Verification items for the finished model (mm, model axes). Give positions to 0.01 mm unless a question says otherwise; leave off trailing zeros. Order: outer loops, then holes, each group sorted by start corner. A loop starts at its lowest first (then second) coordinate and runs counter-clockwise, first axis right, second up. Notation, with made-up numbers: (49.25, 33.5) -> (93.25, 33.5) arc R16 ccw to (93.25, 56.5) -> close; hole circle Ø1 at (48.25, 10.25). An arc over 180 degrees is marked (long way). One line per question, with ' | ' between items. Start each with the question number.
Q1. Material ranges on probe 1 along X at (y, z) = (105.5, 3.5); probe 2 along Y at (x, z) = (-114.3, 5.75); probe 3 along X at (y, z) = (99, 3), recorded low to high. Write a range as [from, to].
Q2. Section check A-A on x = -114.3. Record the cut outline in (y, z), plus the area to 3 significant figures.
Q3. Section check C-C on x = -323.85. Record the cut outline in (y, z).
Q4. Go/stop test with flat-tipped pins: pin 1 (2 mm diameter, centred on x = -303, z = 4, fed in from +Y); pin 2 (1.5 mm diameter, centred on y = 137, z = 5.5, fed in from +X). Record where each tip stops, or that it passes through.
Q5. Section check B-B on y = 29. Record the cut outline in (x, z).
Q6. Mould release check, pull along Y, two halves, no side actions. Record for faces 1 (the cylindrical face through (-80.81, 158.52, 3.76)), 2 (the cylindrical face through (-366.55, 107.02, 3.76)), 3 (the flat face through (-50.57, 25.46, 3.76)): released by +Y, released by -Y, zero draft, split by the parting line, or undercut.
Q7. Section check D-D on z = 2.75. Give the number of separate pieces and of enclosed holes in the cut face, plus the area to 3 significant figures.
from build123d import *

# Parameters (mm, degrees)
SKETCH1_R           = 27.4955
SKETCH1_R_2         = 52.3875
SKETCH1_R_3         = 3.2512
SKETCH1_R_4         = 4.49961
BOSS_EXTRUDE1_DEPTH = 7.62


with BuildPart() as part:
    # Sketch1 → Boss-Extrude1 (new body)
    with BuildSketch(Plane.XY):
        with BuildLine():
            Line((-328.252358788, 147.362734983), (-120.623830303, 167.33652539))
            ThreePointArc((-120.623830303, 167.33652539), (-80.305183306, 158.218318925), (-53.30558743, 126.917251733))
            Line((-53.30558743, 126.917251733), (-9.46754648, 21.302488163))
            ThreePointArc((-9.46754648, 21.302488163), (-11.996916286, 10.47886003), (-23.061809086, 9.422079593))
            Line((-23.061809086, 9.422079593), (-78.866488962, 41.953179506))
            ThreePointArc((-78.866488962, 41.953179506), (-82.120777387, 42.89869406), (-85.437090509, 42.2012285))
            ThreePointArc((-85.437090509, 42.2012285), (-113.899521097, 35.561214301), (-142.440389403, 41.855543485))
            ThreePointArc((-142.440389403, 41.855543485), (-145.776424621, 42.51215325), (-149.027245523, 41.515945031))
            Line((-149.027245523, 41.515945031), (-223.676633484, -3.557736497))
            ThreePointArc((-223.676633484, -3.557736497), (-228.504182895, -4.928354428), (-233.358329437, -3.655134819))
            Line((-233.358329437, -3.655134819), (-346.816870084, 61.773732857))
            ThreePointArc((-346.816870084, 61.773732857), (-368.77925543, 111.345290274), (-328.252358788, 147.362734983))
        make_face()
        with Locations(Location((-323.85, 101.6, 0), (0, 0, 180))):
            Circle(SKETCH1_R, mode=Mode.SUBTRACT)
        with Locations(Location((-114.3, 101.6, 0), (0, 0, 180))):
            Circle(SKETCH1_R_2, mode=Mode.SUBTRACT)
        with Locations(Location((-228.6, 4.596163622, 0), (0, 0, 180))):
            Circle(SKETCH1_R_3, mode=Mode.SUBTRACT)
        with Locations(Location((-18.264817524, 17.65096147, 0), (0, 0, 180))):
            Circle(SKETCH1_R_3, mode=Mode.SUBTRACT)
        with Locations(Location((-323.85, 140.59916, 0), (0, 0, 180))):
            Circle(SKETCH1_R_4, mode=Mode.SUBTRACT)
        with Locations(Location((-298.781823164, 131.475089804, 0), (0, 0, 180))):
            Circle(SKETCH1_R_4, mode=Mode.SUBTRACT)
        with Locations(Location((-285.443324871, 108.372133065, 0), (0, 0, 180))):
            Circle(SKETCH1_R_4, mode=Mode.SUBTRACT)
        with Locations(Location((-290.075736714, 82.10042, 0), (0, 0, 180))):
            Circle(SKETCH1_R_4, mode=Mode.SUBTRACT)
        with Locations(Location((-310.511501707, 64.952777131, 0), (0, 0, 180))):
            Circle(SKETCH1_R_4, mode=Mode.SUBTRACT)
        with Locations(Location((-337.188498293, 64.952777131, 0), (0, 0, 180))):
            Circle(SKETCH1_R_4, mode=Mode.SUBTRACT)
        with Locations(Location((-357.624263286, 82.10042, 0), (0, 0, 180))):
            Circle(SKETCH1_R_4, mode=Mode.SUBTRACT)
        with Locations(Location((-362.256675129, 108.372133065, 0), (0, 0, 180))):
            Circle(SKETCH1_R_4, mode=Mode.SUBTRACT)
        with Locations(Location((-348.918176836, 131.475089804, 0), (0, 0, 180))):
            Circle(SKETCH1_R_4, mode=Mode.SUBTRACT)
    extrude(amount=BOSS_EXTRUDE1_DEPTH)


solid = part.part
Filled in:
1) probe 1: [-369.66, -365.72], [-358.79, -351.07], [-296.63, -288.91], [-281.98, -166.54], [-62.06, -44.42] | probe 2: [35.56, 49.21], [153.99, 167.64] | probe 3: [-369.75, -351.22], [-296.48, -166.62], [-61.98, -41.72]
2) outline: (35.56, 0) -> (49.21, 0) -> (49.21, 7.62) -> (35.56, 7.62) -> close; (153.99, 0) -> (167.64, 0) -> (167.64, 7.62) -> (153.99, 7.62) -> close | area: 208 mm²
3) outline: (48.53, 0) -> (74.1, 0) -> (74.1, 7.62) -> (48.53, 7.62) -> close; (129.1, 0) -> (136.1, 0) -> (136.1, 7.62) -> (129.1, 7.62) -> close; (145.1, 0) -> (147.79, 0) -> (147.79, 7.62) -> (145.1, 7.62) -> close
4) pin 1: y = 149.89 | pin 2: x = -58.08
5) outline: (-289.98, 0) -> (-169.76, 0) -> (-169.76, 7.62) -> (-289.98, 7.62) -> close; (-56.65, 0) -> (-12.66, 0) -> (-12.66, 7.62) -> (-56.65, 7.62) -> close
6) face 1: released by +Y | face 2: undercut | face 3: released by -Y
7) separate pieces: 1 | enclosed holes: 13 | area: 29,900 mm²
